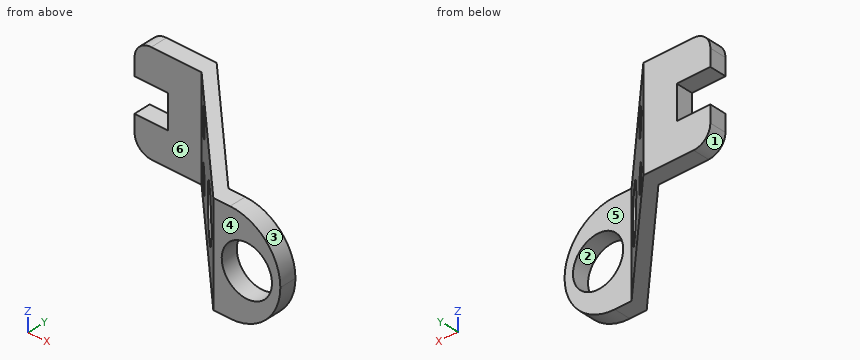
from build123d import *

# Parameters (mm, degrees)
SALIENTE_EXTRUIR1_DEPTH    = 60
CROQUIS3_W                 = 40
CROQUIS3_H                 = 20
CORTAR_EXTRUIR1_DEPTH      = 46
CROQUIS4_R                 = 15
CORTAR_EXTRUIR5_DEPTH      = 57
CORTAR_EXTRUIR6_DEPTH      = 16
CORTAR_EXTRUIR6_DEPTH_BACK = 19
CROQUIS12_R                = 7.5
CROQUIS12_R_2              = 15
REDONDEO2_R                = 10
REDONDEO3_R                = 30


with BuildPart() as part:
    # Croquis2 → Saliente-Extruir1 (new body)
    with BuildSketch(Plane.XY):
        Polygon((-36.180131723, 22.907142857), (3.819868277, 22.907142857), (74.767829948, -48.040818814), (114.767829948, -48.040818814), (114.767829948, -38.040818814), (74.767829948, -38.040818814), (3.819868277, 32.907142857), (-36.180131723, 32.907142857), align=None)
    extrude(amount=SALIENTE_EXTRUIR1_DEPTH)

    # Croquis3 → Cortar-Extruir1 (cut)
    with BuildSketch(Plane(origin=(0, 0, 0), x_dir=(1, 0, 0), z_dir=(0, 1, 0))):
        with Locations((-36.180131723, -30)):
            Rectangle(CROQUIS3_W, CROQUIS3_H)
    extrude(amount=CORTAR_EXTRUIR1_DEPTH, mode=Mode.SUBTRACT)

    # Croquis4 → Cortar-Extruir5 (cut)
    with BuildSketch(Plane(origin=(0, 0, 0), x_dir=(1, 0, 0), z_dir=(0, 1, 0))):
        with Locations(Location((94.767829948, -30, 0), (0, 0, 270))):
            Circle(CROQUIS4_R)
    extrude(amount=-CORTAR_EXTRUIR5_DEPTH, mode=Mode.SUBTRACT)

    # Croquis12 → Cortar-Extruir6 (cut, two sides: drawn at the far end of the back side and taken through both)
    with BuildSketch(Plane(origin=(18.363505567, 18.363505567, 0), x_dir=(0, 0, -1), z_dir=(0.7071067811865486, 0.7071067811865465, 0)).offset(-CORTAR_EXTRUIR6_DEPTH_BACK)):
        with Locations(Location((-15, -4.516083302, 0), (0, 0, 270))):
            Circle(CROQUIS12_R)
        with Locations(Location((-45, -4.516083302, 0), (0, 0, 270))):
            Circle(CROQUIS12_R)
        with Locations(Location((-30, -54.683868112, 0), (0, 0, 270))):
            Circle(CROQUIS12_R_2)
    extrude(amount=CORTAR_EXTRUIR6_DEPTH + CORTAR_EXTRUIR6_DEPTH_BACK, mode=Mode.SUBTRACT)

    # Redondeo2
    redondeo2_edges = [part.edges().sort_by_distance(p)[0] for p in [
        (-36.180131723, 27.907142857, 0),
        (-36.180131723, 27.907142857, 60),
    ]]
    fillet(redondeo2_edges, radius=REDONDEO2_R)

    # Redondeo3
    redondeo3_edges = [part.edges().sort_by_distance(p)[0] for p in [
        (114.767829948, -43.040818814, 60),
        (114.767829948, -43.040818814, 0),
    ]]
    fillet(redondeo3_edges, radius=REDONDEO3_R - 0.0001)  # a hair under: the kernel refuses the full size


solid = part.part
Build history of the part. All positions in model axes, mm. Face numbers are marked on the shaded views. A direction names the side the tool comes from. Coordinates: 2 decimals unless noted, no trailing zeros. Write each loop counter-clockwise with the first axis right and the second up, starting at its lowest first coordinate (ties: lowest second). Pieces come first, ordered by that corner, then holes. Notation, with made-up numbers: (39, -38.5) -> (49, -38.5) arc R16 ccw to (49, -34.5) -> close; hole circle Ø6 at (4, 61.5). An arc over 180 degrees is marked (long way). Use CSV: the item, a comma, the result in double quotes. Start each with the question number.
Q1. Drill centre lines: probe 1 along X at (y, z) = (-40.25, 30); probe 2 along Y at (x, z) = (100, 55.5); probe 3 along X at (y, z) = (-43, 30). Where is each one in solid material? Low to high.
Q2. Flat gauge pins, fed straight in: pin 1 Ø5 at (y, z) = (-27, 9) entering from -X; pin 2 Ø12 at (x, z) = (103.5, 18) entering from +Y; pin 3 Ø3 at (y, z) = (28, 27) entering from -X. Where does each tip first touch, or does it go through?
Q3. Cut at A-A, the plane x = -19.5. List the corners of the cut face in (y, z).
Q4. Cut at C-C, the plane y = 2.5. List the corners of the cut face in (x, z).
Q5. Cut at D-D, the plane x = 73. List the corners of the cut face in (y, z).
Q6. Cut at B-B, the plane z = 35. List the corners of the cut face in (x, y), then the cut area to 3 significant figures.
Q7. Pull direction X, two halves, no side cores. Call the marked faces 1, 2 and 3: released by +X, released by -X, zero draft, split by the parting line, or undercut.
Q8. 3-axis set-ups, long thin cutter, end or side, ignore diameter. For the marked faces 4, 5 and 6: which of +Z, -Z, +X, -X, +Y, -Y reach the whole face in a straight line?
Checked values:
1,probe 1,"x = 66.98 to 79.77, 109.77 to 114.77"
1,probe 2,"y = -48.04 to -38.04"
1,probe 3,"x = 69.73 to 79.77, 109.77 to 114.77"
2,pin 1,"stops at x = 51.23"
2,pin 2,"stops at y = -38.04"
2,pin 3,"stops at x = -16.18"
3,outline,"(22.91, 0) -> (32.91, 0) -> (32.91, 20) -> (22.91, 20) -> close; (22.91, 40) -> (32.91, 40) -> (32.91, 60) -> (22.91, 60) -> close"
4,outline,"(24.23, 0) -> (34.23, 0) -> (34.23, 60) -> (24.23, 60) -> close"
5,outline,"(-46.27, 0) -> (-36.27, 0) -> (-36.27, 60) -> (-46.27, 60) -> close"
6,outline,"(-16.18, 22.91) -> (3.82, 22.91) -> (42.03, -15.3) -> (47.03, -10.3) -> (3.82, 32.91) -> (-16.18, 32.91) -> close; (62.03, -35.3) -> (74.77, -48.04) -> (80.63, -48.04) -> (80.63, -38.04) -> (74.77, -38.04) -> (67.03, -30.3) -> close; (108.91, -48.04) -> (114.35, -48.04) -> (114.35, -38.04) -> (108.91, -38.04) -> close"
6,area,"822 mm²"
7,face 1,"released by -X"
7,face 2,"undercut"
7,face 3,"released by +X"
8,face 4,"+Z, -Z, +X, -X, -Y"
8,face 5,"+Z, -Z, +X, +Y"
8,face 6,"+Z, -Z, -X, -Y"
